The listing builds one solid part. Answer for the finished solid, in the listing's coordinates (mm). A direction names the side the tool comes from. Round coordinates to 2 decimals unless told otherwise and drop trailing zeros. Order: outer loops, then holes, each group sorted by start corner. A loop starts at its lowest first (then second) coordinate and runs counter-clockwise, first axis right, second up. Notation, with made-up numbers: (-19, 41.25) - (-13, 41.25) arc R30 cw to (-13, 69.25) - close; hole circle Ø7 at (19.25, 7). An arc over 180 degrees is marked (long way). Write item = value, one per line.
Autodesk Inventor part; units mm, degrees
ref_plane "Work Plane1" through (0, 0, 2.5) normal (0, 0, 1) x (1, 0, 0)
ref_plane "YZ Plane" through (0, 0, 0) normal (1, 0, 0) x (0, 1, 0)
ref_plane "XZ Plane" through (0, 0, 0) normal (0, 1, 0) x (-1, 0, 0)
sketch "Sketch1" plane through (0, 0, 0) normal (0, 0, 1) x (1, 0, 0)
  line L0 (10, -10) -> (-10, -10)
  line L1 (-10, -10) -> (-10, 10)
  line L2 (-10, 10) -> (10, 10)
  line L3 (10, 10) -> (10, -10)
  line L4 (10, -10) -> (-10, 10) construction
  line L5 (-10, -10) -> (10, 10) construction
  line L6 (10, -10) -> (6, -10)
  line L7 (6, 10) -> (10, 10)
  line L8 (10, 10) -> (10, -10)
  line L9 (0, 10) -> (0, -10)
  line L10 (0, -10) -> (0, 10)
  point P0 (0, 0)
  dimension "d0" = 20
  dimension "d1" = 20
extrude "Extrusion1" add sketch "Sketch1" along normal blind 5 contours L0 L9 L2 L3
ref_plane "Work Plane1" through (0, 0, 2.5) normal (0, 0, 1) x (1, 0, 0)
sketch "Sketch2" plane through (0, 0, 2.5) normal (0, 0, 1) x (1, 0, 0)
  line L0 (0, 10) -> (0, -10)
  line L1 (0, 2.8868) -> (2.5, 1.4434)
  line L2 (2.5, 1.4434) -> (2.5, -1.4434)
  line L3 (2.5, -1.4434) -> (0, -2.8868)
  line L4 (0, -2.8868) -> (-2.5, -1.4434)
  line L5 (-2.5, -1.4434) -> (-2.5, 1.4434)
  line L6 (-2.5, 1.4434) -> (0, 2.8868)
  point P0 (0, 0)
  point P1 (0, 0)
  dimension "d12" = 5
extrude "Extrusion2" cut sketch "Sketch2" along normal mid plane 2
sketch "Sketch3" plane through (0, 0, 5) normal (0, 0, 1) x (1, 0, 0)
  circle A0 centre (0, 0) radius 1.75
  dimension "d15" = 3.5
extrude "Extrusion3" cut sketch "Sketch3" against normal blind 8
sketch "Sketch4" plane through (10, -10, 0) normal (1, 0, 0) x (0, 0, -1)
  circle A0 centre (-2.5, 17.5) radius 1.35
  circle A1 centre (-2.5, 2.5) radius 1.35
  line L0 (0, 20) -> (-5, 20)
  line L1 (0, 0) -> (-5, 0)
  line L2 (0, 0) -> (0, 20)
  point P0 (0, 10)
  dimension "d18" = 2.5
  dimension "d19" = 2.5
  dimension "d20" = 2.5
  dimension "d21" = 2.5
  dimension "d22" = 2.7
  dimension "d23" = 2.7
extrude "Extrusion4" cut sketch "Sketch4" against normal blind 25
sketch "Sketch5" plane through (10, -10, 0) normal (1, 0, 0) x (0, 0, -1)
  circle A0 centre (-2.5, 17.5) radius 1.35
  circle A1 centre (-2.5, 17.5) radius 2
  circle A2 centre (-2.5, 2.5) radius 1.35
  circle A3 centre (-2.5, 2.5) radius 2
  point P0 (0, 10)
  dimension "d26" = 4
  dimension "d27" = 4
extrude "Extrusion5" cut sketch "Sketch5" against normal blind 4 contours A0 | A1 | A2 | A3
sketch "Sketch6" plane through (0, 0, 5) normal (0, 0, 1) x (1, 0, 0)
  point P0 (0, 0)
sketch "Sketch7" plane through (0, 0, 5) normal (0, 0, 1) x (1, 0, 0)
  line L0 (10, -10) -> (10, 10)
  line L1 (10, 10) -> (5, 10)
  line L2 (5, 10) -> (5, 5)
  line L3 (5, 5) -> (10, 5)
  line L4 (10, 5) -> (10, 10)
  line L5 (0, -10) -> (10, -10)
  line L6 (10, -10) -> (5, -10)
  line L7 (5, -10) -> (5, -5)
  line L8 (5, -5) -> (10, -5)
  line L9 (10, -5) -> (10, -10)
  point P0 (0, 0)
  dimension "d30" = 5
  dimension "d31" = 5
  dimension "d32" = 5
  dimension "d33" = 5
extrude "Extrusion6" cut sketch "Sketch7" against normal blind 10
sketch "Sketch8" plane through (10, -5, 0) normal (1, 0, 0) x (0, 0, -1)
  line L0 (0, 0) -> (5, 0)
  line L1 (5, 0) -> (5, 10)
  line L2 (5, 10) -> (0, 10)
  line L3 (0, 10) -> (0, 0)
  line L4 (-5, 0) -> (-5, 10)
  line L5 (-5, 10) -> (-10, 10)
  line L6 (-10, 10) -> (-10, 0)
  line L7 (-10, 0) -> (-5, 0)
  line L8 (-5, 0) -> (-5, 10)
  circle A0 centre (-7.5, 5) radius 1.35
  circle A1 centre (2.5, 5) radius 1.35
  point P0 (0, 5)
  point P1 (-7.5, 0)
  dimension "d36" = 5
  dimension "d37" = 5
  dimension "d38" = 5
  dimension "d39" = 2.7
  dimension "d40" = 2.7
  dimension "d41" = 5
  dimension "d42" = 5
  dimension "d43" = 5
  dimension "d44" = 5
  dimension "d45" = 2.5
  dimension "d46" = 2.5
extrude "Extrusion7" add sketch "Sketch8" against normal blind 5
sketch "Sketch9" plane through (5, -5, 0) normal (-1, 0, 0) x (0, 0, 1)
  circle A0 centre (7.5, 5) radius 1.35
  circle A1 centre (7.5, 5) radius 2
  circle A2 centre (-2.5, 5) radius 1.35
  circle A3 centre (-2.5, 5) radius 2
  point P0 (0, 5)
  dimension "d49" = 4
  dimension "d50" = 4
extrude "Extrusion8" cut sketch "Sketch9" against normal blind 2 contours A0 | A1 | A2 | A3
sketch "Sketch10" plane through (5, 10, 5) normal (1, 0, 0) x (0, 0, -1)
  circle A0 centre (2.5, -2.5) radius 1.35
  circle A1 centre (2.5, -2.5) radius 2.35
  circle A2 centre (2.5, -17.5) radius 1.35
  circle A3 centre (2.5, -17.5) radius 2.35
  point P0 (5, -10)
  dimension "d53" = 4.7
  dimension "d54" = 4.7
extrude "Extrusion9" cut sketch "Sketch10" against normal blind 2.6
equation "\"d18\" = d19"
equation "\"d20\" = d19"
equation "\"d21\" = d19"
equation "\"d23\" = d22"
equation "\"d27\" = d26"
equation "\"d39\" = d40"
equation "\"d42\" = d41"
equation "\"d50\" = d49"
properties part number "POMSliderMotor" material "Acetal Resin, White"
Q1. Section B-B on y = 7.5 is taken. Determine the outline of the cut face in (x, z), then the cut area to 3 significant figures.
Model answer:
outline = (0, 0) - (5, 0) - (5, 0.15) - (2.4, 0.15) - (2.4, 1.15) - (0, 1.15) - close; (0, 3.85) - (2.4, 3.85) - (2.4, 4.85) - (5, 4.85) - (5, 5) - (0, 5) - close
area = 6.30 mm^2
Q2. For faces 1 (the face through (5.986, -1.952, -2.934)), 2 (the face through (5, 2.3, 7.5)), 3 (the face through (5, 2.3, -2.5)), determine the directions among +Z, -Z, +X, -X, +Y, -Y from which every point of the face is accessible in a straight line to the end or side of a thin tool.
Model answer:
face_1 = -X
face_2 = +Z, -X, +Y, -Y
face_3 = -Z, -X, +Y, -Y
Q3. Section A-A on z = 2.5 is taken. Determine the outline of the cut face in (x, y), then the cut area to 3 significant figures.
Model answer:
outline = (0, -10) - (5, -10) - (5, -9.85) - (2.4, -9.85) - (2.4, -8.85) - (0, -8.85) - close; (0, -6.15) - (2.4, -6.15) - (2.4, -5.15) - (5, -5.15) - (5, -5) - (10, -5) - (10, 5) - (5, 5) - (5, 5.15) - (2.4, 5.15) - (2.4, 6.15) - (0, 6.15) - (0, 2.89) - (2.5, 1.44) - (2.5, -1.44) - (0, -2.89) - close; (0, 8.85) - (2.4, 8.85) - (2.4, 9.85) - (5, 9.85) - (5, 10) - (0, 10) - close
area = 102 mm^2
Q4. Find the intervals of material crossed by line 1 (Y direction, x = 4.2, z = 2.5); line 2 (Y direction, x = 8.5, z = -1.5); line 3 (Z direction, x = 3.5, y = 3.5), in increasing order. Write a range as from..to.
Model answer:
line_1 = -10..-9.85, -5.15..5.15, 9.85..10
line_2 = -5..-0.91, 0.91..5
line_3 = 0..5
Q5. Determine the mould class of faces 4 (the face through (8.521, 0.406, 6.212)), 5 (the face through (7, -5, 3)), 6 (the face through (2, 0, 0)) for opening direction Y: released by +Y, released by -Y, zero draft, split by the parting line, or undercut.
Model answer:
face_4 = undercut
face_5 = released by -Y
face_6 = zero draft
Q6. Section D-D on y = 0 is taken. Determine the outline of the cut face in (x, z), then the cut area to 4 significant figures.
Model answer:
outline = (1.75, 0) - (5, 0) - (5, -0.5) - (7, -0.5) - (7, -1.15) - (10, -1.15) - (10, 6.15) - (7, 6.15) - (7, 5.5) - (5, 5.5) - (5, 5) - (1.75, 5) - (1.75, 3.5) - (2.5, 3.5) - (2.5, 1.5) - (1.75, 1.5) - close; (5, -5) - (10, -5) - (10, -3.85) - (7, -3.85) - (7, -4.5) - (5, -4.5) - close; (5, 9.5) - (7, 9.5) - (7, 8.85) - (10, 8.85) - (10, 10) - (5, 10) - close
area = 57.55 mm^2
Q7. Flat-ended cylindrical pins translate along their axes: P1, Ø3, axis at y = 0, z = 7.5, coming from the -X side; P2, Ø4, axis at y = -7.5, z = 3, coming from the +X side; P3, Ø2, axis at y = 0, z = 3, coming from the -X side; P4, Ø3, axis at y = 0, z = -2.5, coming from the +X side. Find the tip coordinate at first contact, or state that the pin passes through.
Model answer:
P1 = 7
P2 = 5
P3 = 1.52
P4 = 10
Q8. Section C-C on z = 7.5 is taken. Determine the outline of the cut face in (x, y).
Model answer:
outline = (5, -5) - (10, -5) - (10, -1.35) - (7, -1.35) - (7, -2) - (5, -2) - close; (5, 2) - (7, 2) - (7, 1.35) - (10, 1.35) - (10, 5) - (5, 5) - close
